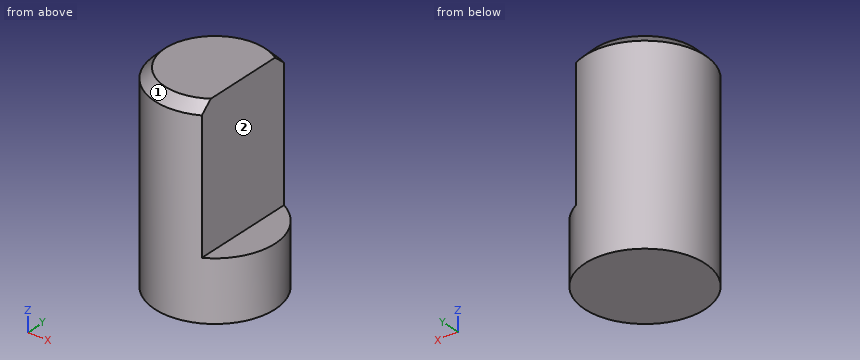
from build123d import *

# Parameters (mm, degrees)
BOX009_W          = 6
BOX009_H          = 6
BOX009_DEPTH      = 7
CYLINDER001_R     = 3
CYLINDER001_DEPTH = 10
CHAMFER002_SIZE   = 0.5


with BuildPart() as rotary_top_cutout:
    # Box009 → Box009 (new body)
    with BuildSketch(Plane(origin=(1.4, -3, 3), x_dir=(1, 0, 0), z_dir=(0, 0, 1))):
        with Locations((3, 3)):
            Rectangle(BOX009_W, BOX009_H)
    extrude(amount=BOX009_DEPTH)


with BuildPart() as chamfer002:
    # Cylinder001 → Cylinder001 (new body)
    with BuildSketch(Plane.XY):
        Circle(CYLINDER001_R)
    extrude(amount=CYLINDER001_DEPTH)

    # Cut017: cut ROTARY_top_cutout
    add(rotary_top_cutout.part, mode=Mode.SUBTRACT)

    # Chamfer002
    chamfer002_edges = [chamfer002.edges().sort_by_distance(p)[0] for p in [
        (-3, 0, 10),
    ]]
    chamfer(chamfer002_edges, length=CHAMFER002_SIZE)


solid = chamfer002.part
Geometry: final body of the model. Coordinates: model frame, mm. Face numbers are marked on the shaded views. A direction names the side the tool comes from. Give positions to 0.01 mm unless a question says otherwise; leave off trailing zeros. Loops run counter-clockwise (first coordinate to the right, second up) from the corner with the lowest first, then second, coordinate; pieces in that order, holes last. Notation, with made-up numbers: M -13,-13.75 L 23,-13.75 A8 cw 23,-9.75 Z; hole C 55.5,65.25 d7. An arc over 180 degrees is marked long. Put each result on its own line as item: value.
1) Cut plane A-A, the plane y = 0. Return the cut outline in (x, z), plus the area to 3 significant figures.
Computed values:
outline: M -3,0 L 3,0 L 3,3 L 1.4,3 L 1.4,10 L -2.5,10 L -3,9.5 Z
area: 48.7 mm^2
2) First-contact query: P1, Ø0.8, axis at x = 2, y = -1, coming from the +Z side. Flat tip, straight axial feed; report the tip coordinate or a pass-through.
Computed values:
P1: stops at z = 3
3) Reachability of the marked faces 1 and 2 from +Z, -Z, +X, -X, +Y, -Y: full face, straight path, thin tool, end or side. Return the list, or none.
Computed values:
face 1: +Z
face 2: +Z, +X, +Y, -Y
4) Cut plane D-D, the plane z = 4.75. Return the cut outline in (x, y).
Computed values:
outline: M 1.4,-2.65 L 1.4,2.65 A3 ccw long Z
5) Cut plane C-C, the plane x = 2. Return the cut outline in (y, z), plus the area to 3 significant figures.
Computed values:
outline: M -2.24,0 L 2.24,0 L 2.24,3 L -2.24,3 Z
area: 13.4 mm^2
6) Material intervals for L1, parallel to Z at x = 2.05, y = 1.4; L2, parallel to Y at x = 0.6, z = 6; L3, parallel to Y at x = 1.1, z = 4.5, sorted ascending. Write a range as from..to.
Computed values:
L1: z = 0..3
L2: y = -2.94..2.94
L3: y = -2.79..2.79
7) Cut plane B-B, the plane z = 1.75. Return the cut outline in (x, y).
Computed values:
outline: C 0,0 d6
